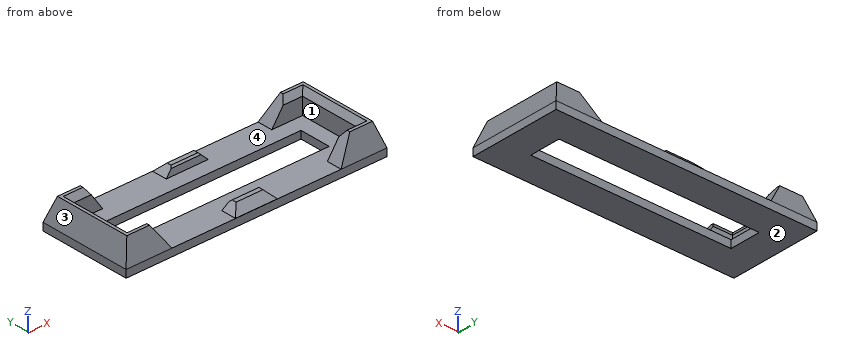
```python
from build123d import *

# Parameters (mm, degrees)
F0_W      = 172
F0_H      = 60.5
F4_DEPTH  = 5
F6_SIZE2  = 4
F6_SIZE   = 3
F9_DEPTH  = 5
F10_SIZE  = 4.99999
F11_SIZE2 = 0.99999
F11_SIZE  = 4.99999
F12_SIZE  = 1
F14_W     = 132
F14_H     = 20.5
F15_DEPTH = 12.5


# Not quite as in the source:
# - a fillet or chamfer is up to 0.001 mm smaller than in the source, because OpenCascade refuses the exact size


with BuildPart() as f4:
    # F0 (on Top) → F4 (new body)
    with BuildSketch(Plane.XY):
        Rectangle(F0_W, F0_H)
    extrude(amount=-F4_DEPTH)

    # F3 (on Top) → F5 section 0
    with BuildSketch(Plane.XY):
        Polygon((-86, 0), (-86, -30.25), (-55.75, -30.25), (-55.75, -20.25), (-76, -20.25), (-76, 0), align=None)
    # F2 (on offset) → F5 section 1
    with BuildSketch(Plane.XY.offset(15)):
        Polygon((-76, -20.25), (-76, 0), (-81, 0), (-81, -25.25), (-66, -25.25), (-66, -20.25), align=None)
    loft()

    # F6
    f6_edges = [f4.edges().sort_by_distance(p)[0] for p in [
        (-76, -10.125, 15),
        (-71, -20.25, 15),
    ]]
    chamfer(f6_edges, length=F6_SIZE, length2=F6_SIZE2)

    # F7: F4 across plane


with BuildPart() as f4_1:
    add(f4.part)
    add(f4.part.mirror(Plane.YZ))

    # F8 (on face) → F9 (join)
    with BuildSketch(Plane.XY):
        Polygon((13.8189587742, -20.25), (0, -20.25), (-13.8189587742, -20.25), (-13.8189587742, -30.1344580948), (0, -30.1344580948), (13.8189587742, -30.1344580948), align=None)
    extrude(amount=F9_DEPTH)

    # F10 (size 5 in the source; OpenCascade refuses exactly that, so slightly less here)
    f10_edges = [f4_1.edges().sort_by_distance(p)[0] for p in [
        (13.818959, -25.192229, 5),
        (0, -30.134458, 5),
        (-13.818959, -25.192229, 5),
    ]]
    chamfer(f10_edges, length=F10_SIZE)

    # F11 (size 5 and 1 in the source; OpenCascade refuses exactly that, so slightly less here)
    f11_edges = [f4_1.edges().sort_by_distance(p)[0] for p in [
        (0, -20.25, 5),
    ]]
    f11_side = f4_1.faces().sort_by_distance((0, -20.25, 2.315943))[0]
    chamfer(f11_edges, length=F11_SIZE, length2=F11_SIZE2, reference=f11_side)

    # F12
    f12_edges = [f4_1.edges().sort_by_distance(p)[0] for p in [
        (0, -21.24999, 5),
    ]]
    chamfer(f12_edges, length=F12_SIZE)

    # F13: F4 across plane


with BuildPart() as f4_2:
    add(f4_1.part)
    add(f4_1.part.mirror(Plane.XZ))

    # F14 (on Top) → F15 (cut, symmetric)
    with BuildSketch(Plane.XY):
        Rectangle(F14_W, F14_H)
    extrude(amount=F15_DEPTH, both=True, mode=Mode.SUBTRACT)


solid = f4_2.part
```
CAD build for the part. Positions are in the model's coordinates, mm. Face numbers are marked on the shaded views. Give positions to 0.01 mm unless a question says otherwise; leave off trailing zeros. Loops run counter-clockwise (first coordinate to the right, second up) from the corner with the lowest first, then second, coordinate; pieces in that order, holes last. Notation, with made-up numbers: (-30, -14) -> (-17, -14) arc R14 ccw to (-17, -8) -> close; hole circle Ø5 at (49.25, 59). An arc over 180 degrees is marked (long way). Use a Markdown table: item, result.
1. Flat gauge pins, fed straight in: pin 1 (5 mm diameter, centred on y = 0.5, z = 2, fed in from +X); pin 2 (2 mm diameter, centred on y = 3, z = 4.5, fed in from -X); pin 3 (3 mm diameter, centred on x = -4, y = -23, fed in from +Z); pin 4 (3 mm diameter, centred on y = -17.5, z = 9, fed in from +X). Where does each tip first touch, or does it go through?
Check result:
| item | result |
|---|---|
| pin 1 | stops at x = 86 |
| pin 2 | stops at x = -84.83 |
| pin 3 | stops at z = 5 |
| pin 4 | stops at x = 83.5 |
2. Slice it at D-D (y = -12). List the corners of the cut face in (x, z), plus the area to 3 significant figures.
Check result:
| item | result |
|---|---|
| outline | (-86, -5) -> (86, -5) -> (86, 0) -> (81, 15) -> (79, 15) -> (76, 11) -> (76, 0) -> (-76, 0) -> (-76, 11) -> (-79, 15) -> (-81, 15) -> (-86, 0) -> close |
| area | 1,070 mm^2 |
3. Wall check: L1, parallel to Y at x = 61.5, z = 0.25; L2, parallel to Y at x = 32, z = -3.75; L3, parallel to Z at x = 50, y = 19. Give the ranges that are in metal, low to high. Write a range as [from, to].
Check result:
| item | result |
|---|---|
| L1 | y = [-30.17, -20.25], [20.25, 30.17] |
| L2 | y = [-30.25, -10.25], [10.25, 30.25] |
| L3 | z = [-5, 0] |
4. Mould opens along X. For the marked faces 1, 2, 3 and 4 say: pulls with the +X half, pulls with the -X half, needs draft (parallel to the pull), parting line crosses it, or undercut.
Check result:
| item | result |
|---|---|
| face 1 | undercut |
| face 2 | needs draft |
| face 3 | pulls with the -X half |
| face 4 | undercut |
5. Slice it at A-A (y = 2). List the corners of the cut face in (x, z).
Check result:
| item | result |
|---|---|
| outline | (-86, -5) -> (-66, -5) -> (-66, 0) -> (-76, 0) -> (-76, 11) -> (-79, 15) -> (-81, 15) -> (-86, 0) -> close; (66, -5) -> (86, -5) -> (86, 0) -> (81, 15) -> (79, 15) -> (76, 11) -> (76, 0) -> (66, 0) -> close |
6. Slice it at C-C (z = -2.5). List the corners of the cut face in (x, y), plus the area to 3 significant figures.
Check result:
| item | result |
|---|---|
| outline | (-86, -30.25) -> (86, -30.25) -> (86, 30.25) -> (-86, 30.25) -> close; hole (-66, -10.25) -> (66, -10.25) -> (66, 10.25) -> (-66, 10.25) -> close |
| area | 7,700 mm^2 |
7. Slice it at B-B (x = 19.5). List the corners of the cut face in (y, z), plus the area to 3 significant figures.
Check result:
| item | result |
|---|---|
| outline | (-30.25, -5) -> (-10.25, -5) -> (-10.25, 0) -> (-30.25, 0) -> close; (10.25, -5) -> (30.25, -5) -> (30.25, 0) -> (10.25, 0) -> close |
| area | 200 mm^2 |
